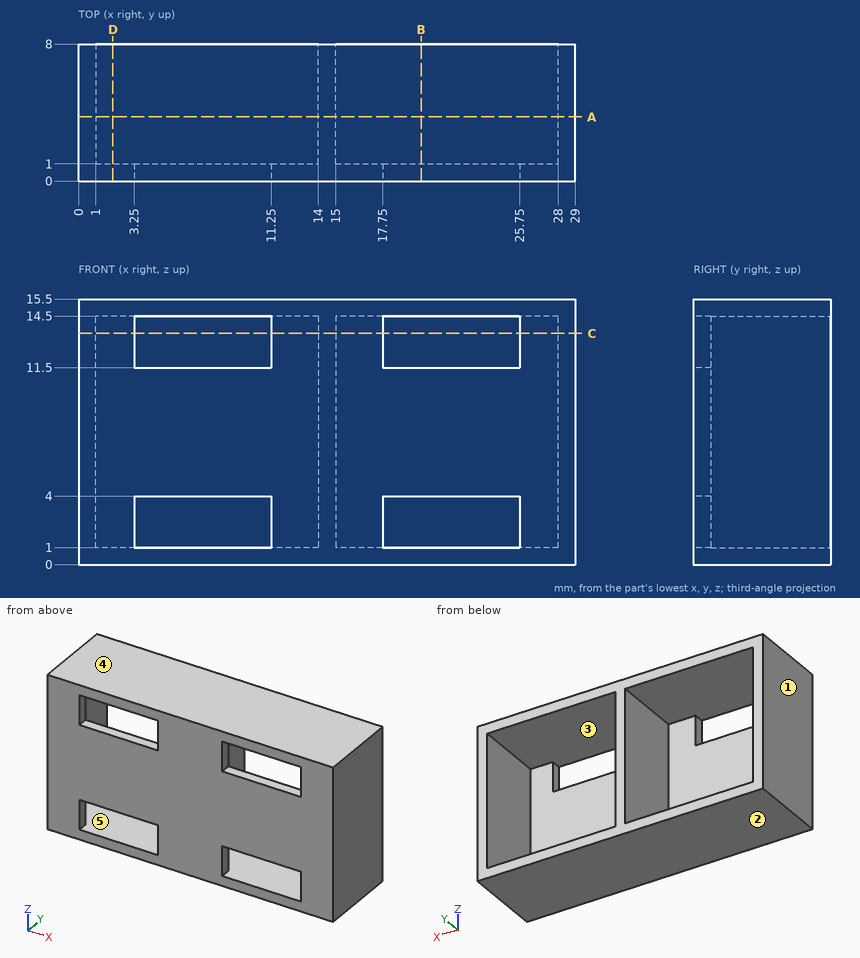
For this review, use the dimensioned drawing (mm, ordinates from the lowest corner) and the shaded views. A direction names the side the tool comes from. Coordinates: 2 decimals unless noted, no trailing zeros. Write each loop counter-clockwise with the first axis right and the second up, starting at its lowest first coordinate (ties: lowest second). Pieces come first, ordered by that corner, then holes. Notation, with made-up numbers: (61, 85) -> (80, 85) arc R30 ccw to (80, 108) -> close; hole circle Ø4 at (18.5, -25). An arc over 180 degrees is marked (long way). Write each question's results on one line, items separated by ' | '. Start each with the question number.
(1) For line 1 along X through (y, z) = (4, 13.75); line 2 along Z through (x, y) = (23.5, 1.5); line 3 along X through (y, z) = (0.75, 2), list the stretches that pass through material, from the lowest coordinate up. Write a range as from..to.
(2) Take a section at D-D on x = 2. Write out the cut boundary in (y, z), and give its area (3 significant figures).
(3) Take a section at A-A on y = 3.75. Write out the cut boundary in (x, z), and give its area (3 significant figures).
(4) Tool access review of the marked faces 4 and 5: name each direction out of +Z, -Z, +X, -X, +Y, -Y from which nothing blocks a thin tool from reaching the whole face with its end or side.
(5) Take a section at B-B on x = 20. Write out the cut boundary in (y, z).
(6) Clearance check with flat-ended pins moving along their axes: P1, Ø4, axis at x = 24.5, z = 10.5, coming from the -Y side; P2, Ø1, axis at x = 8, z = 13.5, coming from the -Y side; P3, Ø4, axis at x = 20.5, z = 8, coming from the +Y side. State where each tip first meets the part, or that it passes through.
(7) The part is to be moulded in two halves that separate along X. For the marked faces 1, 2 and 3, say which applies: pulls with the +X half, pulls with the -X half, needs draft (parallel to the pull), parting line crosses it, or undercut.
(8) Take a section at C-C on z = 13.5. Write out the cut boundary in (x, y), and give its area (3 significant figures).
Results found:
1) line 1: x = 0..1, 14..15, 28..29 | line 2: z = 0..1, 14.5..15.5 | line 3: x = 0..3.25, 11.25..17.75, 25.75..29
2) outline: (0, 0) -> (8, 0) -> (8, 1) -> (1, 1) -> (1, 14.5) -> (8, 14.5) -> (8, 15.5) -> (0, 15.5) -> close | area: 29.5 mm2
3) outline: (0, 0) -> (29, 0) -> (29, 15.5) -> (0, 15.5) -> close; hole (1, 1) -> (14, 1) -> (14, 14.5) -> (1, 14.5) -> close; hole (15, 1) -> (28, 1) -> (28, 14.5) -> (15, 14.5) -> close | area: 98.5 mm2
4) face 4: +Z, +X, -X, +Y, -Y | face 5: +Y
5) outline: (0, 0) -> (8, 0) -> (8, 1) -> (0, 1) -> close; (0, 4) -> (1, 4) -> (1, 11.5) -> (0, 11.5) -> close; (0, 14.5) -> (8, 14.5) -> (8, 15.5) -> (0, 15.5) -> close
6) P1: stops at y = 0 | P2: passes through | P3: stops at y = 1
7) face 1: pulls with the -X half | face 2: needs draft | face 3: undercut
8) outline: (0, 0) -> (3.25, 0) -> (3.25, 1) -> (1, 1) -> (1, 8) -> (0, 8) -> close; (11.25, 0) -> (17.75, 0) -> (17.75, 1) -> (15, 1) -> (15, 8) -> (14, 8) -> (14, 1) -> (11.25, 1) -> close; (25.75, 0) -> (29, 0) -> (29, 8) -> (28, 8) -> (28, 1) -> (25.75, 1) -> close | area: 34.0 mm2
